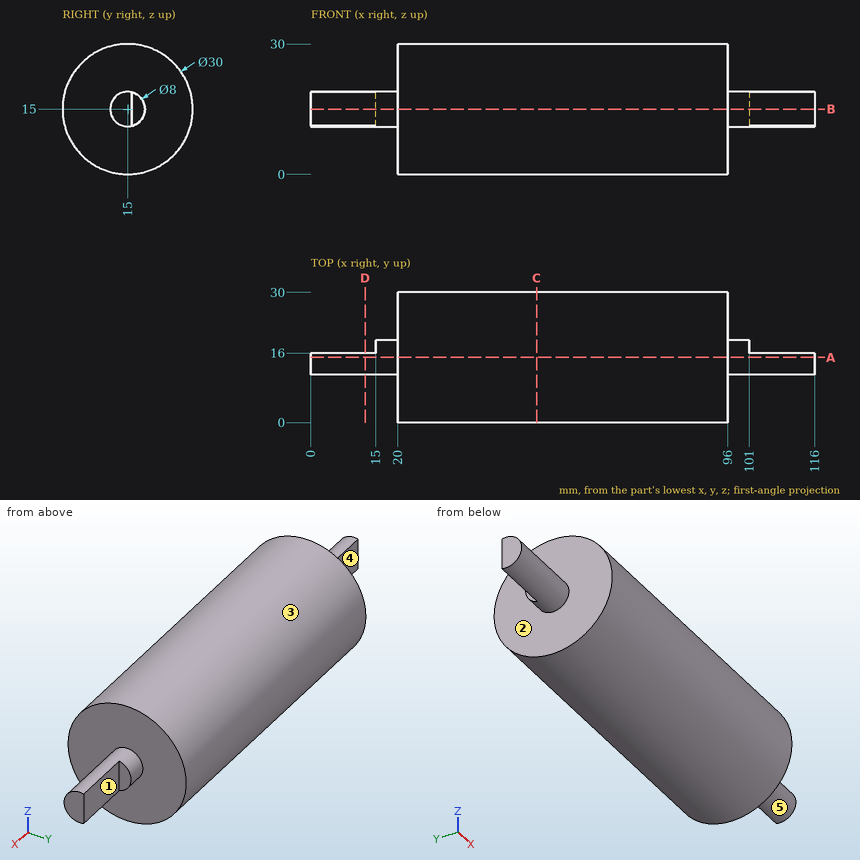
Geometry check sheet. Reference: drawing and pictorial views, mm from the part's lowest x, y, z. A direction names the side the tool comes from. Give positions to 0.01 mm unless a question says otherwise; leave off trailing zeros. Order: outer loops, then holes, each group sorted by start corner. A loop starts at its lowest first (then second) coordinate and runs counter-clockwise, first axis right, second up. Notation, with made-up numbers: M 9.5,78.25 L 19.5,78.25 A26 cw 19.5,96.25 Z; hole C 59,-33 d3. An arc over 180 degrees is marked long. Use one line per item in the form item = value. Start each with the question number.
Q1. Section check C-C (x = 52). Enter the section's corners in (y, z).
Q2. Section check D-D (x = 12.5). Enter the section's corners in (y, z).
Q3. Section check B-B (z = 15). Enter the section's corners in (x, y).
Q4. Access from +Z, -Z, +X, -X, +Y, -Y to the whole of each face (thin tool, end or side, straight path). Record for the marked faces 1, 2, 3, 4 and 5.
Q5. Section check A-A (y = 15). Enter the section's corners in (x, z).
Q6. Scan lines: line 1 along Z through (x, y) = (78.5, 14.5); line 2 along X through (y, z) = (26, 13.5); line 3 along Z through (x, y) = (84, 20.75). Record each from-to range of solid material in increasing order. Write a range as [from, to].
Q7. Go/stop test with flat-tipped pins: pin 1 Ø12 at (y, z) = (22, 10.5) entering from -X; pin 2 Ø8.5 at (x, z) = (11, 15.5) entering from +Y; pin 3 Ø4 at (x, z) = (100.5, 7.5) entering from -Y; pin 4 Ø8 at (x, y) = (84.5, 5.5) entering from -Z. Record where each tip stops, or that it passes through.
Evaluation:
q1.outline = C 15,15 d30
q2.outline = M 16,11.13 L 16,18.87 A4 ccw long Z
q3.outline = M 0,11 L 20,11 L 20,0 L 96,0 L 96,11 L 116,11 L 116,16 L 101,16 L 101,19 L 96,19 L 96,30 L 20,30 L 20,19 L 15,19 L 15,16 L 0,16 Z
q4.face_1 = +Z, -Z, +X, +Y
q4.face_2 = -X
q4.face_3 = +X, -X
q4.face_4 = +Z, -Z, -X, +Y
q4.face_5 = +X
q5.outline = M 0,11 L 20,11 L 20,0 L 96,0 L 96,11 L 116,11 L 116,19 L 96,19 L 96,30 L 20,30 L 20,19 L 0,19 Z
q6.line_1 = [0.01, 29.99]
q6.line_2 = [20, 96]
q6.line_3 = [1.15, 28.85]
q7.pin_1 = 15
q7.pin_2 = 19
q7.pin_3 = through
q7.pin_4 = 1.04
